```python
from build123d import *

# Parameters (mm, degrees)
F_1P5MM_12_DEPTH            = 12
CUT_EXTRUDE_M3_DEPTH        = 100
CUT_EXTRUDE_M3_DEPTH_BACK   = 100
SKETCH_2_R                  = 1.6
CUT_EXTRUDE_M3_2_DEPTH      = 100
CUT_EXTRUDE_M3_2_DEPTH_BACK = 100
SKETCH_3_R                  = 1.6


with BuildPart() as part:
    # 草图1 → 1p5mm直角固定座_宽12 (new body)
    with BuildSketch(Plane.XY):
        Polygon((-5, 0), (12.5, 0), (12.5, -10), (14, -10), (14, 1.5), (-5, 1.5), align=None)
    extrude(amount=F_1P5MM_12_DEPTH)

    # 草图2 → Cut-Extrude M3 (cut, two sides: drawn at the far end of the back side and taken through both)
    with BuildSketch(Plane(origin=(0, 0, 0), x_dir=(1, 0, 0), z_dir=(0, 1, 0)).offset(-CUT_EXTRUDE_M3_DEPTH_BACK)):
        with Locations(Location((0, -6, 0), (0, 0, 270))):
            Circle(SKETCH_2_R)
    extrude(amount=CUT_EXTRUDE_M3_DEPTH + CUT_EXTRUDE_M3_DEPTH_BACK, mode=Mode.SUBTRACT)

    # 草图3 → Cut-Extrude M3 2 (cut, two sides: drawn at the far end of the back side and taken through both)
    with BuildSketch(Plane(origin=(0, 0, 0), x_dir=(0, 0, -1), z_dir=(1, 0, 0)).offset(-CUT_EXTRUDE_M3_2_DEPTH_BACK)):
        with Locations((-6, -5)):
            Circle(SKETCH_3_R)
    extrude(amount=CUT_EXTRUDE_M3_2_DEPTH + CUT_EXTRUDE_M3_2_DEPTH_BACK, mode=Mode.SUBTRACT)


solid = part.part
```
Can you work these out from the model? Positions are in its coordinate system, mm. A direction names the side the tool comes from. Round coordinates to 2 decimals unless told otherwise and drop trailing zeros. Loops run counter-clockwise (first coordinate to the right, second up) from the corner with the lowest first, then second, coordinate; pieces in that order, holes last.
Item 1: Suppose I cut it at D-D, the plane z = 9. Write out the boundary of the cut face in (x, y).
Item 2: Please list where these lines run through material, in increasing order: L1, parallel to X at y = 0.6, z = 6; L2, parallel to Z at x = 0, y = 0.6; L3, parallel to X at y = -5, z = 2.5.
Item 3: Suppose I cut it at B-B, the plane y = -5. Write out the boundary of the cut face in (x, z).
Item 4: Suppose I cut it at A-A, the plane x = 0. Write out the boundary of the cut face in (y, z).
Item 5: Suppose I cut it at C-C, the plane z = 6. Write out the boundary of the cut face in (x, y), then the cut area to 3 significant figures.
Item 6: Which directions (+Z, -Z, +X, -X, +Y, -Y) give clear straight access to the entire face, cutting with the end or side of a thin tool? Please do faces 1 (the flat face through (13, -10, 6)), 2 (the flat face through (12.5, -6.04, 4.58)).
Item 7: If we mould it in two halves opening along Z, with no side actions, what happens to faces 3 (the flat face through (5, 1.5, 6)), 4 (the cylindrical face through (0.481, 0.74, 7.526)), 5 (the flat face through (6.6, 0.5, 0)), 6 (the flat face through (6.6, 0.5, 12))? For each: +Z half, -Z half, draft (parallel to the pull), parting line (faces both ways), or undercut.
Item 8: Will these pins go through, and if not, where does the flat tip stop? pin 1 Ø2 at (x, y) = (5, -2.5) entering from -Z; pin 2 Ø3 at (y, z) = (-3, 4.5) entering from -X.
Reported:
1. outline: (-5, 0) - (12.5, 0) - (12.5, -10) - (14, -10) - (14, 1.5) - (-5, 1.5) - close
2. L1: x = -5 to -1.6, 1.6 to 14
2. L2: z = 0 to 4.4, 7.6 to 12
2. L3: x = 12.5 to 14
3. outline: (12.5, 0) - (14, 0) - (14, 4.4) - (12.5, 4.4) - close; (12.5, 7.6) - (14, 7.6) - (14, 12) - (12.5, 12) - close
4. outline: (0, 0) - (1.5, 0) - (1.5, 4.4) - (0, 4.4) - close; (0, 7.6) - (1.5, 7.6) - (1.5, 12) - (0, 12) - close
5. outline: (-5, 0) - (-1.6, 0) - (-1.6, 1.5) - (-5, 1.5) - close; (1.6, 0) - (12.5, 0) - (12.5, -3.4) - (14, -3.4) - (14, 1.5) - (1.6, 1.5) - close; (12.5, -10) - (14, -10) - (14, -6.6) - (12.5, -6.6) - close
5. area: 33.9 mm2
6. face 1: +Z, -Z, +X, -X, -Y
6. face 2: +Z, -Z, -X, -Y
7. face 3: draft
7. face 4: undercut
7. face 5: -Z half
7. face 6: +Z half
8. pin 1: passes through
8. pin 2: stops at x = 12.5
